from build123d import *

# Parameters (mm, degrees)
F0_W        = 140
F0_H        = 252.5
F0_R        = 1
F0_W_2      = 94
F0_H_2      = 152.5
F0_R_2      = 2.5
F0_W_3      = 12
F0_H_3      = 34
F1_DEPTH    = 15.56
F2_DEPTH    = 10.56
F3_T1_DEPTH = 165.7168298797
F3_T3_DEPTH = 278.2168298797
F4_SIZE     = 2.5
F5_R        = 3
F6_DEPTH    = 10
F7_SIZE     = 4.99999
F8_W        = 161.2529857084
F8_H        = 70
F9_DEPTH    = 25
F11_W       = 5
F11_H       = 50
F12_DEPTH   = 5


# Not quite as in the source:
# - a fillet or chamfer that OpenCascade refuses, or shapes differently, is made with other operations: its cross-section is extruded or revolved along the edge and cut away or added
# - a fillet or chamfer is up to 0.001 mm smaller than in the source, because OpenCascade refuses the exact size
# - a feature names something its author has since deleted; it is built from what else it names


with BuildPart() as f1:
    # F0 (on Front) → F1 (new body)
    with BuildSketch(Plane.XZ):
        with Locations((-70, 126.25)):
            Rectangle(F0_W, F0_H)
        with Locations((-135, 5)):
            Circle(F0_R, mode=Mode.SUBTRACT)
        with Locations((-5, 5)):
            Circle(F0_R, mode=Mode.SUBTRACT)
        with Locations((-135, 247.5)):
            Circle(F0_R, mode=Mode.SUBTRACT)
        Polygon((-130, 44), (-130, 242.5), (-10, 242.5), (-10, 44), (-64, 44), (-64, 10), (-76, 10), (-76, 44), align=None, mode=Mode.SUBTRACT)
        with Locations((-5, 247.5)):
            Circle(F0_R, mode=Mode.SUBTRACT)
        Polygon((-10, 242.5), (-130, 242.5), (-130, 44), (-76, 44), (-64, 44), (-10, 44), align=None)
        with Locations((-70, 143.25)):
            Rectangle(F0_W_2, F0_H_2, mode=Mode.SUBTRACT)
        with Locations((-70, 232.5)):
            Circle(F0_R_2, mode=Mode.SUBTRACT)
        with Locations((-70, 27)):
            Rectangle(F0_W_3, F0_H_3)
    extrude(amount=F1_DEPTH)

    # F0 (on Front) → F2 (cut)
    with BuildSketch(Plane.XZ):
        Polygon((-10, 242.5), (-130, 242.5), (-130, 44), (-76, 44), (-64, 44), (-10, 44), align=None)
        with Locations((-70, 143.25)):
            Rectangle(F0_W_2, F0_H_2, mode=Mode.SUBTRACT)
        with Locations((-70, 232.5)):
            Circle(F0_R_2, mode=Mode.SUBTRACT)
        with Locations((-70, 27)):
            Rectangle(F0_W_3, F0_H_3)
    extrude(amount=F2_DEPTH, mode=Mode.SUBTRACT)

    # F3: chamfer of 5 on 4 edges, made by hand

    # F3_s2 → F3_t1 (cut)
    with BuildSketch(Plane.YZ.offset(-152.8584149398)):
        Polygon((-10.56, 0), (-15.56, 5), (-15.56, 0), align=None)
        Polygon((-15.56, 247.5), (-10.56, 252.5), (-15.56, 252.5), align=None)
    extrude(amount=F3_T1_DEPTH, mode=Mode.SUBTRACT)

    # F3_s4 → F3_t3 (cut)
    with BuildSketch(Plane.XY.offset(-12.8584149398)):
        Polygon((-140, -10.56), (-135, -15.56), (-140, -15.56), align=None)
        Polygon((0, -10.56), (-5, -15.56), (0, -15.56), align=None)
    extrude(amount=F3_T3_DEPTH, mode=Mode.SUBTRACT)

    # F4
    f4_edges = [f1.edges().sort_by_distance(p)[0] for p in [
        (-72.5, -15.56, 232.5),
    ]]
    chamfer(f4_edges, length=F4_SIZE)

    # F5 (on face) → F6 (cut)
    with BuildSketch(Plane.XZ.offset(15.56)):
        with Locations((-135, 247.5)):
            Circle(F5_R)
        with Locations((-135, 5)):
            Circle(F5_R)
        with Locations((-5, 247.5)):
            Circle(F5_R)
        with Locations((-5, 5)):
            Circle(F5_R)
    extrude(amount=-F6_DEPTH, mode=Mode.SUBTRACT)

    # F7 (size 5 in the source; OpenCascade refuses exactly that, so slightly less here)
    f7_edges = [f1.edges().sort_by_distance(p)[0] for p in [
        (-70, -15.56, 67),
        (-117, -15.56, 143.25),
        (-23, -15.56, 143.25),
        (-70, -15.56, 219.5),
    ]]
    chamfer(f7_edges, length=F7_SIZE)

    # F8 (on face) → F9 (cut)
    with BuildSketch(Plane.XZ.offset(15.56)):
        with Locations((-74.815297965, 217.5)):
            Rectangle(F8_W, F8_H)
    extrude(amount=-F9_DEPTH, mode=Mode.SUBTRACT)

    # F11 (on offset) → F12 (join)
    with BuildSketch(Plane(origin=(0, -2.5, 0), x_dir=(-1, 0, 0), z_dir=(0, 1, 0))):
        with Locations((135, 182.5)):
            Rectangle(F11_W, F11_H)
        with Locations((5, 182.5)):
            Rectangle(F11_W, F11_H)
    extrude(amount=-F12_DEPTH)


solid = f1.part
Geometry check sheet. Reference: the model listing, model coordinates, mm. A direction names the side the tool comes from. Round coordinates to 2 decimals unless told otherwise and drop trailing zeros. Order: outer loops, then holes, each group sorted by start corner. A loop starts at its lowest first (then second) coordinate and runs counter-clockwise, first axis right, second up. Notation, with made-up numbers: M -0.5,82 L 7.5,82 A24 cw 7.5,98 Z; hole C -2.75,-2 d3. An arc over 180 degrees is marked long. Answer in a Markdown table with one row per item.
(1) Scan lines: probe 1 along X at (y, z) = (-1.9, 5); probe 2 along Z at (x, y) = (-135, -8.25); probe 3 along X at (y, z) = (-6.25, 82.5). Record each from-to range of solid material in increasing order. Write a range as from..to.
Responses:
| item | result |
|---|---|
| probe 1 | x = -140..-136, -134..-6, -4..0 |
| probe 2 | z = 0..2, 8..182.5 |
| probe 3 | x = -140..-130, -10..0 |
(2) Sectioned sample at B-B, the plane z = 49.5. Record the cut outline in (x, y).
Responses:
| item | result |
|---|---|
| outline | M -140,-10.56 L -135,-15.56 L -5,-15.56 L 0,-10.56 L 0,0 L -10,0 L -10,-10.56 L -130,-10.56 L -130,0 L -140,0 Z |
(3) Draft check along X on faces 4 (the face through (-76, -5, 27)), 5 (the face through (-5, -2.5, 195)), 6 (the face through (0, -5, 90)). Enter one of: released by +X, released by -X, zero draft, split by the parting line, or undercut.
Responses:
| item | result |
|---|---|
| face 4 | undercut |
| face 5 | zero draft |
| face 6 | released by +X |
(4) Tool access check on faces 1 (the face through (-70.728, -13.025, 64.535)), 2 (the face through (-37, -5, 44)), 3 (the face through (-136, -5.56, 6)). Record the directions out of +Z, -Z, +X, -X, +Y, -Y that give a thin tool (end or side, any length) a straight path to the whole face; none if there is none.
Responses:
| item | result |
|---|---|
| face 1 | +Z, -Y |
| face 2 | +Z, +Y |
| face 3 | -Y |
(5) Go/stop test with flat-tipped pins: P1, Ø4, axis at y = -4.5, z = 191.5, coming from the +X side; P2, Ø4, axis at y = -4.5, z = 189.5, coming from the -X side; P3, Ø5.5, axis at x = -73, y = -5, coming from the +Z side. Record where each tip stops, or that it passes through.
Responses:
| item | result |
|---|---|
| P1 | stops at x = -2.5 |
| P2 | stops at x = -137.5 |
| P3 | stops at z = 10 |
